from build123d import *

# Parameters (mm, degrees)
SKETCH_1_R          = 2
EXTRUDE_1_DEPTH     = 13
SKETCH_2_W          = 7
SKETCH_2_H          = 34.84138361
CUT_EXTRUDE_1_DEPTH = 193.919672403
SKETCH_3_W          = 10
SKETCH_3_H          = 7
EXTRUDE_2_DEPTH     = 70


with BuildPart() as part:
    # 草图1 → 凸台-拉伸1 (new body)
    with BuildSketch(Plane.XY):
        with BuildLine():
            Line((54, -72), (75, -72))
            ThreePointArc((75, -72), (78.535533906, -73.464466094), (80, -77))
            Line((80, -77), (80, -107))
            Line((80, -107), (-80, -107))
            Line((-80, -107), (-80, -77))
            ThreePointArc((-80, -77), (-78.535533906, -73.464466094), (-75, -72))
            Line((-75, -72), (-54, -72))
            ThreePointArc((-54, -72), (0, -90), (54, -72))
        make_face()
        with Locations(Location((-64.83247643, -87, 0), (0, 0, 180))):
            Circle(SKETCH_1_R, mode=Mode.SUBTRACT)
        with Locations(Location((64.83247643, -87, 0), (0, 0, 180))):
            Circle(SKETCH_1_R, mode=Mode.SUBTRACT)
    extrude(amount=EXTRUDE_1_DEPTH)

    # 草图2 → 切除-拉伸1 (cut, through all)
    with BuildSketch(Plane(origin=(80, 0, 0), x_dir=(0, 0, -1), z_dir=(1, 0, 0))):
        with Locations((-6.5, -87.579308195)):
            Rectangle(SKETCH_2_W, SKETCH_2_H)
    extrude(amount=-CUT_EXTRUDE_1_DEPTH, mode=Mode.SUBTRACT)

    # 草图3 → 凸台-拉伸2 (add)
    with BuildSketch(Plane.XY.offset(13)):
        with Locations((-64.83247643, -103.5)):
            Rectangle(SKETCH_3_W, SKETCH_3_H)
        with Locations((64.83247643, -103.5)):
            Rectangle(SKETCH_3_W, SKETCH_3_H)
    extrude(amount=EXTRUDE_2_DEPTH)


solid = part.part
Read the model definition and answer for the solid it produces. Units are mm, in the model's axes. A direction names the side the tool comes from. Round coordinates to 2 decimals unless told otherwise and drop trailing zeros. Order: outer loops, then holes, each group sorted by start corner. A loop starts at its lowest first (then second) coordinate and runs counter-clockwise, first axis right, second up.
1) Flat-ended cylindrical pins translate along their axes: pin 1 (2 mm diameter, centred on y = -104.5, z = 45, fed in from -X); pin 2 (3 mm diameter, centred on x = 20, y = -87.5, fed in from +Z); pin 3 (8 mm diameter, centred on x = -64.5, z = 38.5, fed in from +Y). Find the tip coordinate at first contact, or state that the pin passes through.
2) Straight lines are drawn through the part: L1, parallel to Z at x = -13, y = -91.5; L2, parallel to X at y = -103, z = 56; L3, parallel to Y at x = -2.5, z = 6. For each, find the intervals that lie inside material, in ascending order.
3) The part is cut by section A-A on y = -101.5. Write down the section's boundary in (x, z), plus the area to 3 significant figures.
4) The mould has two halves that part along Z. Classify faces 1 (the face through (1, -92, 3)), 2 (the face through (78, -73, 11)), 3 (the face through (1, -93, 0)): released by +Z, released by -Z, zero draft, split by the parting line, or undercut.
5) The part is cut by section B-B on y = -87. Give the number of separate pieces and of enclosed holes in the cut face, plus the area to 3 significant figures.
6) The part is cut by section C-C on x = 7. Write down the section's boundary in (y, z).
7) For faces 4 (the face through (59.832, -104, 48)), 5 (the face through (78, -73, 1)), 6 (the face through (80, -92, 11)), 7 (the face through (65, -100, 48)), 8 (the face through (1, -92, 10)), determine the directions among +Z, -Z, +X, -X, +Y, -Y from which every point of the face is accessible in a straight line to the end or side of a thin tool.
8) The part is cut by section D-D on x = -50.5. Write down the section's boundary in (y, z).
Resolved:
1. pin 1: stops at x = -69.83
1. pin 2: stops at z = 13
1. pin 3: stops at y = -100
2. L1: z = 0 to 3, 10 to 13
2. L2: x = -69.83 to -59.83, 59.83 to 69.83
2. L3: y = -107 to -105
3. outline: (-80, 0) - (80, 0) - (80, 3) - (-80, 3) - close; (-80, 10) - (80, 10) - (80, 13) - (69.83, 13) - (69.83, 83) - (59.83, 83) - (59.83, 13) - (-59.83, 13) - (-59.83, 83) - (-69.83, 83) - (-69.83, 13) - (-80, 13) - close
3. area: 2,360 mm2
4. face 1: undercut
4. face 2: zero draft
4. face 3: released by -Z
5. separate pieces: 8
5. enclosed holes: 0
5. area: 635 mm2
6. outline: (-107, 0) - (-89.73, 0) - (-89.73, 3) - (-105, 3) - (-105, 10) - (-89.73, 10) - (-89.73, 13) - (-107, 13) - close
7. face 4: +Z, +Y, -Y
7. face 5: +Z, -Z, +X, +Y
7. face 6: +Z, -Z, +X, +Y, -Y
7. face 7: +Z, +X, -X, +Y
7. face 8: +X, -X, +Y
8. outline: (-107, 0) - (-74.5, 0) - (-74.5, 3) - (-105, 3) - (-105, 10) - (-74.5, 10) - (-74.5, 13) - (-107, 13) - close
